The model under review builds one solid part; all positions refer to its coordinate system, in mm. Face numbers are marked on the shaded views. Coordinates: 2 decimals unless noted, no trailing zeros. Loops run counter-clockwise (first coordinate to the right, second up) from the corner with the lowest first, then second, coordinate; pieces in that order, holes last. Notation, with made-up numbers: M 54.25,73 L 73.25,73 A23 cw 73.25,99 Z; hole C 22.25,-3.5 d4. An arc over 180 degrees is marked long. Return JSON: item names as keys, results as strings.
Autodesk Inventor part; units mm, degrees
ref_plane "YZ Plane" through (0, 0, 0) normal (1, 0, 0) x (0, 1, 0)
ref_plane "XZ Plane" through (0, 0, 0) normal (0, 1, 0) x (-1, 0, 0)
ref_plane "XY Plane" through (0, 0, 0) normal (0, 0, 1) x (1, 0, 0)
sketch "Sketch1" plane through (0, 0, 0) normal (0, 0, 1) x (1, 0, 0)
  circle A0 centre (0, 0) radius 100 construction
  circle A1 centre (0, 0) radius 100.1
  circle A2 centre (0, 0) radius 102.1
  point P0 (0, 0)
  dimension "d0" = 0.1
  dimension "d1" = 2
extrude "Extrusion1" add sketch "Sketch1" against normal blind 15
sketch "Sketch2" plane through (0, 0, 0) normal (0, 0, 1) x (1, 0, 0)
  circle A0 centre (0, 0) radius 102.1
  point P0 (0, 0)
extrude "Extrusion2" add sketch "Sketch2" along normal blind 2
fillet "Fillet1" radius 1 1 edges at (-102.1, 0, -15)
fillet "Fillet1" radius 2 1 edges at (-102.1, 0, 2)
properties part number "cap_v2"
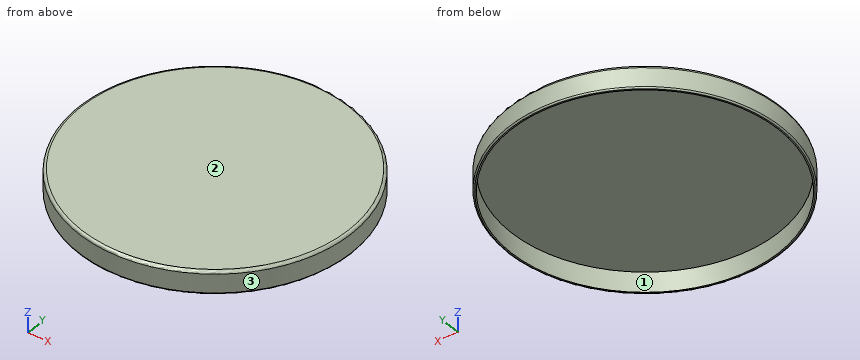
1. The part is to be moulded in two halves that separate along Y. For the marked faces 1, 2 and 3, say which applies: released by +Y, released by -Y, zero draft, split by the parting line, or undercut.
Check values:
{"face 1": "undercut", "face 2": "zero draft", "face 3": "split by the parting line"}
2. To check wall thickness, follow line 1 (Y direction, x = 0, z = -9); line 2 (Z direction, x = 82, y = -13.5); line 3 (Y direction, x = -8, z = -5.75). State the ranges of each line that lie inside material, in increasing order.
Check values:
{"line 1": "-102.1 to -100.1, 100.1 to 102.1", "line 2": "0 to 2", "line 3": "-101.79 to -99.78, 99.78 to 101.79"}
3. Add section C-C on z = -2.5. Give the boundary of the cut face in (x, y).
Check values:
{"outline": "C 0,0 d204.2; hole C 0,0 d200.2"}
4. Add section A-A on x = 0. Give the boundary of the cut face in (y, z), plus the area to 3 significant figures.
Check values:
{"outline": "M -102.1,-14 A1 ccw -101.1,-15 L -100.1,-15 L -100.1,0 L 100.1,0 L 100.1,-15 L 101.1,-15 A1 ccw 102.1,-14 L 102.1,0 A2 ccw 100.1,2 L -100.1,2 A2 ccw -102.1,0 Z", "area": "466 mm²"}
5. Insertion check: pin 1 Ø1 at (x, z) = (46, -1.5) entering from +Y; pin 2 Ø1.5 at (x, y) = (-18.5, -53.5) entering from -Z; pin 3 Ø6 at (x, z) = (-58.5, -10) entering from -Y. Each pin has a flat end and moves straight along its axis. Give the tip position at first contact, or say it passes through.
Check values:
{"pin 1": "y = 91.4", "pin 2": "z = 0", "pin 3": "y = -85.7"}
